```python
from build123d import *

# Parameters (mm, degrees)
F0_W      = 76.2
F0_H      = 76.2
F1_DEPTH  = 50.8
F2_W      = 25.4
F2_H      = 76.2
F3_DEPTH  = 12.7
F6_W      = 26.153776
F6_H      = 25.4
F7_DEPTH  = 25.4
F5_W      = 50.453637
F5_H      = 25.4
F8_DEPTH  = 25.4
F9_W      = 25.4
F9_H      = 12.7
F10_DEPTH = 25.4
F11_W     = 25.4
F11_H     = 12.7
F12_DEPTH = 25.4
F14_D     = 12.7


with BuildPart() as f1:
    # F0 (on Top) → F1 (new body)
    with BuildSketch(Plane.XY):
        Rectangle(F0_W, F0_H)
    extrude(amount=F1_DEPTH)

    # F2 (on face) → F3 (cut)
    with BuildSketch(Plane.XY.offset(50.8)):
        Rectangle(F2_W, F2_H)
    extrude(amount=-F3_DEPTH, mode=Mode.SUBTRACT)

    # F6 (on face) → F7 (cut)
    with BuildSketch(Plane(origin=(0, 0, 0), x_dir=(1, 0, 0), z_dir=(0, 0, -1))):
        with Locations((-25.776888, 0.036548)):
            Rectangle(F6_W, F6_H)
    extrude(amount=-F7_DEPTH, mode=Mode.SUBTRACT)

    # F5 (on face) → F8 (cut)
    with BuildSketch(Plane(origin=(0, 0, 0), x_dir=(1, 0, 0), z_dir=(0, 0, -1))):
        with Locations((12.526818, -0.04948)):
            Rectangle(F5_W, F5_H)
    extrude(amount=-F8_DEPTH, mode=Mode.SUBTRACT)

    # F9 (on face) → F10 (cut)
    with BuildSketch(Plane.YZ.offset(38.1)):
        with Locations((0, 6.35)):
            Rectangle(F9_W, F9_H)
    extrude(amount=-F10_DEPTH, mode=Mode.SUBTRACT)

    # F11 (on face) → F12 (cut)
    with BuildSketch(Plane.YZ.offset(38.1)):
        with Locations((0, 19.05)):
            Rectangle(F11_W, F11_H)
    extrude(amount=-F12_DEPTH, mode=Mode.SUBTRACT)

    # F14 (through all)
    with Locations(Plane.XY.offset(38.1)):
        with Locations((0, 0)):
            Hole(F14_D / 2)


solid = f1.part
```
For this review, take the finished solid that the model builds, in its own axes (mm). A direction names the side the tool comes from. Round coordinates to 2 decimals unless told otherwise and drop trailing zeros. Write each loop counter-clockwise with the first axis right and the second up, starting at its lowest first coordinate (ties: lowest second). Pieces come first, ordered by that corner, then holes.
1) Insertion check: pin 1 Ø12 at (x, y) = (19, 5) entering from -Z; pin 2 Ø16.5 at (x, y) = (0, 0) entering from +Z. Each pin has a flat end and moves straight along its axis. Give the tip position at first contact, or say it passes through.
Answer below:
pin 1: stops at z = 25.4
pin 2: stops at z = 38.1
2) For line 1 along Y through (x, z) = (0, 28); line 2 along X through (y, z) = (-14.5, 44); line 3 along Y through (x, z) = (21, 7), list the stretches that pass through material, from the lowest coordinate up.
Answer below:
line 1: y = -38.1 to -6.35, 6.35 to 38.1
line 2: x = -38.1 to -12.7, 12.7 to 38.1
line 3: y = -38.1 to -12.7, 12.75 to 38.1
3) Mouldability with a two-part tool opening along X and no side actions: class faces 1 (the face through (12.7, -1, 45)), 2 (the face through (-1, -38.1, 25)), 3 (the face through (38.1, -1, 31)) as +X half, -X half, draft (parallel to the pull), parting line (faces both ways), or undercut.
Answer below:
face 1: undercut
face 2: draft
face 3: +X half
4) Take a section at D-D on y = -11.5. Give the boundary of the cut face in (x, z).
Answer below:
outline: (-38.1, 25.4) - (38.1, 25.4) - (38.1, 50.8) - (12.7, 50.8) - (12.7, 38.1) - (-12.7, 38.1) - (-12.7, 50.8) - (-38.1, 50.8) - close
5) Take a section at B-B on z = 42. Give the boundary of the cut face in (x, y), then the cut area to 3 significant figures.
Answer below:
outline: (-38.1, -38.1) - (-12.7, -38.1) - (-12.7, 38.1) - (-38.1, 38.1) - close; (12.7, -38.1) - (38.1, -38.1) - (38.1, 38.1) - (12.7, 38.1) - close
area: 3,870 mm2
6) Take a section at C-C on x = 0. Give the boundary of the cut face in (y, z), then the cut area to 3 significant figures.
Answer below:
outline: (-38.1, 0) - (-12.65, 0) - (-12.65, 25.4) - (-6.35, 25.4) - (-6.35, 38.1) - (-38.1, 38.1) - close; (6.35, 25.4) - (12.75, 25.4) - (12.75, 0) - (38.1, 0) - (38.1, 38.1) - (6.35, 38.1) - close
area: 2,100 mm2
7) Take a section at A-A on y = 0. Give the boundary of the cut face in (x, z), then the cut area to 3 significant figures.
Answer below:
outline: (-38.1, 25.4) - (-6.35, 25.4) - (-6.35, 38.1) - (-12.7, 38.1) - (-12.7, 50.8) - (-38.1, 50.8) - close; (6.35, 25.4) - (38.1, 25.4) - (38.1, 50.8) - (12.7, 50.8) - (12.7, 38.1) - (6.35, 38.1) - close
area: 1,450 mm2
8) Machinability: for faces 4 (the face through (0, -12.651, 13)), 5 (the face through (-1, 38.1, 25)), 6 (the face through (-26, -12.737, 13)), 7 (the face through (-12.7, -1, 45)), which of the approach directions +Z, -Z, +X, -X, +Y, -Y give a long, thin tool a straight path to every point of the face, cutting with its end or side? Answer none if there is none.
Answer below:
face 4: -Z, +X, -X
face 5: +Z, -Z, +X, -X, +Y
face 6: -Z, -X
face 7: +Z, +Y, -Y
